Check sheet for the drawn part. Datum: minimum x, y, z corner. Units: mm. A direction names the side the tool comes from. Round coordinates to 2 decimals unless told otherwise and drop trailing zeros. Order: outer loops, then holes, each group sorted by start corner. A loop starts at its lowest first (then second) coordinate and runs counter-clockwise, first axis right, second up. Notation, with made-up numbers: (-20.75, 88) -> (-3.75, 88) arc R13 ccw to (-3.75, 108) -> close; hole circle Ø11 at (61.5, 74). An arc over 180 degrees is marked (long way). Write item = value, one per line. Start each with the question number.
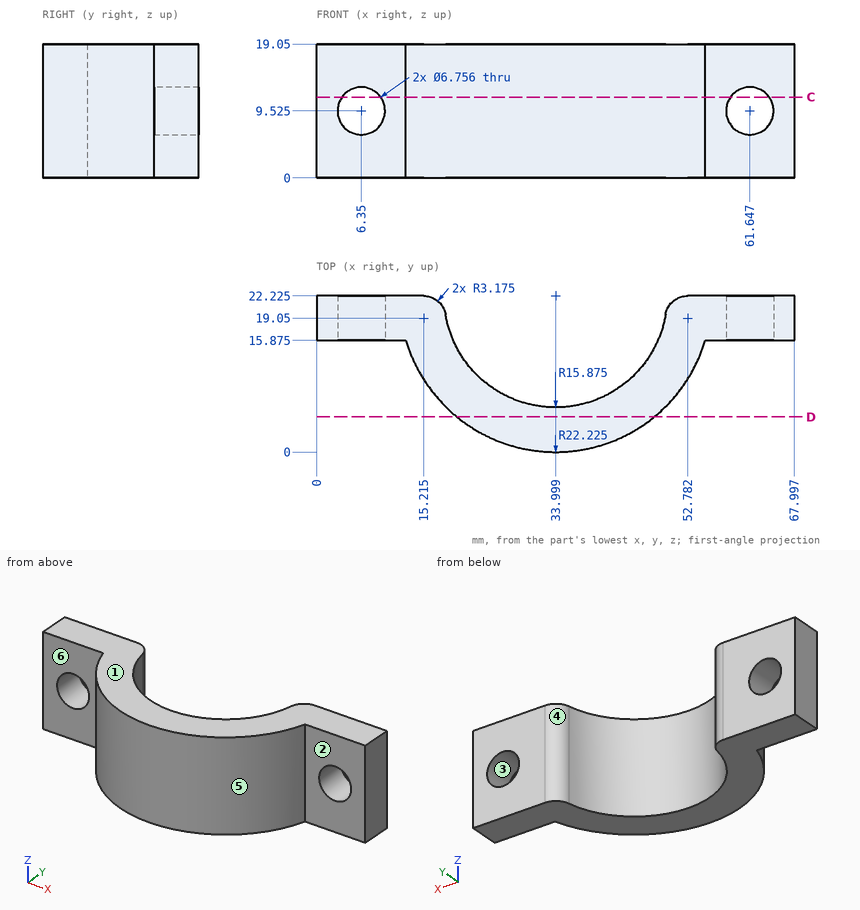
(1) Depth check by flat-ended pin: pin 1 (8 mm diameter, centred on x = 6.35, z = 9.525, fed in from -Y) (3 decimals); pin 2 (1 mm diameter, centred on x = 52, z = 14.5, fed in from +Y); pin 3 (1 mm diameter, centred on x = 33.5, z = 2, fed in from +Y); pin 4 (1.5 mm diameter, centred on x = 10, y = 13.5, fed in from +Z). Enter the tip coordinate at first touch or a pass-through.
(2) Scan lines: line 1 along X through (y, z) = (15.25, 15) (1 decimal); line 2 along X through (y, z) = (21.25, 4.25) (1 decimal); line 3 along Y through (x, z) = (61, 16.75) (1 decimal). Record each from-to range of solid material in increasing order. Write a range as from..to.
(3) Cross-section at D-D (y = 5). Enter the section's corners in (x, z).
(4) Draft check along Z on the marked faces 1, 2 and 3. Enter one of: +Z half, -Z half, draft (parallel to the pull), parting line (faces both ways), or undercut.
(5) Cross-section at C-C (z = 11.5). Give the number of separate pieces and of enclosed holes in the cut face.
(6) Set-up check for the marked faces 4, 5 and 6: record each of +Z, -Z, +X, -X, +Y, -Y from which the full face is reachable in a straight line by a thin tool's end or side.
Outcome:
q1.pin_1 = 15.875
q1.pin_2 = 22.21
q1.pin_3 = 6.38
q1.pin_4 = through
q2.line_1 = 12.9..19.7, 48.3..55.1
q2.line_2 = 0..17.5, 50.5..68
q2.line_3 = 15.9..22.2
q3.outline = (19.95, 0) -> (48.04, 0) -> (48.04, 19.05) -> (19.95, 19.05) -> close
q4.face_1 = +Z half
q4.face_2 = draft
q4.face_3 = undercut
q5.separate_pieces = 3
q5.enclosed_holes = 0
q6.face_4 = +Z, -Z, +Y
q6.face_5 = +Z, -Z, -Y
q6.face_6 = +Z, -Z, -X, -Y
